The listing builds one solid part. Answer for the finished solid, in the listing's coordinates (mm). Face numbers are marked on the shaded views. A direction names the side the tool comes from. Coordinates: 2 decimals unless noted, no trailing zeros. Order: outer loops, then holes, each group sorted by start corner. A loop starts at its lowest first (then second) coordinate and runs counter-clockwise, first axis right, second up. Notation, with made-up numbers: (-33, 76) -> (21, 76) arc R25 ccw to (21, 113) -> close; hole circle Ø7 at (-39.75, 49). An arc over 180 degrees is marked (long way). Return JSON: item names as keys, results as strings.
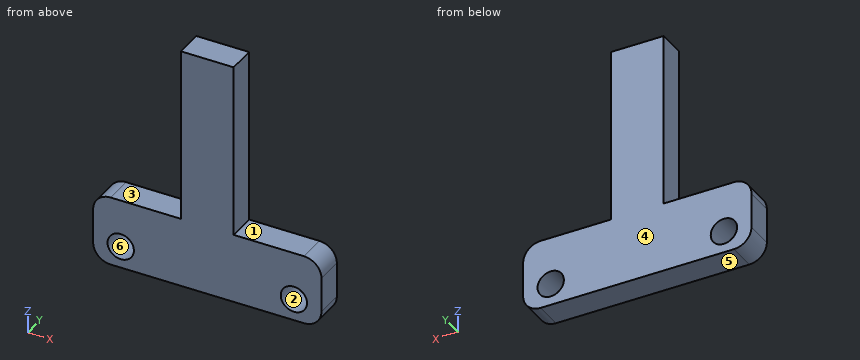
```python
from build123d import *

# Parameters (mm, degrees)
SKETCH_1_R      = 1.5
EXTRUDE_1_DEPTH = 3.175


with BuildPart() as part:
    # 草图1 → 凸台-拉伸1 (new body)
    with BuildSketch(Plane(origin=(0, 0, 0), x_dir=(1, 0, 0), z_dir=(0, 1, 0))):
        with BuildLine():
            Line((-11, 4), (11, 4))
            ThreePointArc((11, 4), (12.414213562, 3.414213562), (13, 2))
            Line((13, 2), (13, -2))
            ThreePointArc((13, -2), (12.414213562, -3.414213562), (11, -4))
            Line((11, -4), (3, -4))
            Line((3, -4), (3, -24))
            Line((3, -24), (-3, -24))
            Line((-3, -24), (-3, -4))
            Line((-3, -4), (-11, -4))
            ThreePointArc((-11, -4), (-12.414213562, -3.414213562), (-13, -2))
            Line((-13, -2), (-13, 2))
            ThreePointArc((-13, 2), (-12.414213562, 3.414213562), (-11, 4))
        make_face()
        with Locations((-9.86, 1.5)):
            Circle(SKETCH_1_R, mode=Mode.SUBTRACT)
        with Locations((9.86, 1.5)):
            Circle(SKETCH_1_R, mode=Mode.SUBTRACT)
    extrude(amount=EXTRUDE_1_DEPTH)


solid = part.part
```
Item 1: Determine the mould class of the marked faces 4, 5 and 6 for opening direction Z: pulls with the +Z half, pulls with the -Z half, needs draft (parallel to the pull), parting line crosses it, or undercut.
Answer list:
{"face 4": "needs draft", "face 5": "pulls with the -Z half", "face 6": "undercut"}
Item 2: The part is cut by section A-A on x = 9.86. Determine the outline of the cut face in (y, z) (3 decimals).
Answer list:
{"outline": "(0, -4) -> (3.175, -4) -> (3.175, -3) -> (0, -3) -> close; (0, 0) -> (3.175, 0) -> (3.175, 4) -> (0, 4) -> close"}
Item 3: Which of the six approach directions +Z, -Z, +X, -X, +Y, -Y give full straight-line access (tool end or side, diameter ignored) to the marked faces 1, 2 and 3?
Answer list:
{"face 1": "+Z, +X, +Y, -Y", "face 2": "+Y, -Y", "face 3": "+Z, -X, +Y, -Y"}
Item 4: The part is cut by section D-D on x = -3.5. Determine the outline of the cut face in (y, z) (3 decimals).
Answer list:
{"outline": "(0, -4) -> (3.175, -4) -> (3.175, 4) -> (0, 4) -> close"}
Item 5: The part is cut by section C-C on y = 1.7. Determine the outline of the cut face in (x, z), plus the area to 3 significant figures.
Answer list:
{"outline": "(-13, -2) arc R2 ccw to (-11, -4) -> (11, -4) arc R2 ccw to (13, -2) -> (13, 2) arc R2 ccw to (11, 4) -> (3, 4) -> (3, 24) -> (-3, 24) -> (-3, 4) -> (-11, 4) arc R2 ccw to (-13, 2) -> close; hole circle Ø3 at (-9.86, -1.5); hole circle Ø3 at (9.86, -1.5)", "area": "310 mm2"}
Item 6: Find the intervals of material crossed by probe 1 along X at (y, z) = (1.45, -1.5); probe 2 along Z at (x, y) = (-9.86, 1.6); probe 3 along X at (y, z) = (1.55, -1), in increasing order.
Answer list:
{"probe 1": "-13 to -11.36, -8.36 to 8.36, 11.36 to 13", "probe 2": "-4 to -3, 0 to 4", "probe 3": "-13 to -11.27, -8.45 to 8.45, 11.27 to 13"}
Item 7: The part is cut by section B-B on z = -1.5. Determine the outline of the cut face in (x, y) (3 decimals).
Answer list:
{"outline": "(-13, 0) -> (-11.36, 0) -> (-11.36, 3.175) -> (-13, 3.175) -> close; (-8.36, 0) -> (8.36, 0) -> (8.36, 3.175) -> (-8.36, 3.175) -> close; (11.36, 0) -> (13, 0) -> (13, 3.175) -> (11.36, 3.175) -> close"}
Item 8: Flat-ended cylindrical pins translate along their axes: pin 1 (1.6 mm diameter, centred on y = 2.5, z = 16, fed in from -X); pin 2 (12 mm diameter, centred on x = 10, z = 17.5, fed in from -Y); pin 3 (1 mm diameter, centred on x = 6.5, y = 1.5, fed in from +Z). Find the tip coordinate at first contact, or state that the pin passes through.
Answer list:
{"pin 1": "x = -3", "pin 2": "through", "pin 3": "z = 4"}
